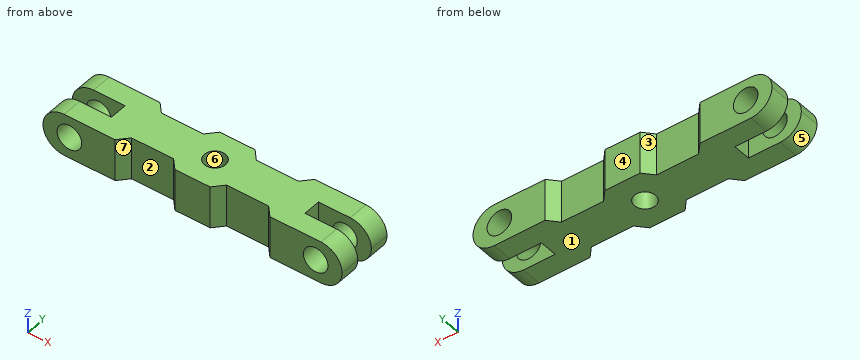
from build123d import *

# Parameters (mm, degrees)
F1_DEPTH = 12
F2_R     = 6
F3_DEPTH = 25
F4_R     = 7
F5_DEPTH = 50
F6_R     = 11.99999
F7_R     = 11.99999


# Not quite as in the source:
# - a fillet or chamfer is up to 0.001 mm smaller than in the source, because OpenCascade refuses the exact size


with BuildPart() as f1:
    # F0 (on Top) → F1 (new body, symmetric)
    with BuildSketch(Plane.XY):
        Polygon((10, 16.5), (0, 16.5), (-10, 16.5), (-15, 11), (-39, 11), (-44, 16.5), (-85, 16.5), (-85, 5), (-55, 5), (-55, 0), (-55, -5), (-85, -5), (-85, -16.5), (-44, -16.5), (-39, -11), (-15, -11), (-10, -16.5), (0, -16.5), (10, -16.5), (15, -11), (39, -11), (44, -16.5), (85, -16.5), (85, -5), (55, -5), (55, 0), (55, 5), (85, 5), (85, 16.5), (44, 16.5), (39, 11), (15, 11), align=None)
    extrude(amount=F1_DEPTH, both=True)

    # F2 (on Top) → F3 (cut, symmetric)
    with BuildSketch(Plane.XY):
        Circle(F2_R)
    extrude(amount=F3_DEPTH, both=True, mode=Mode.SUBTRACT)

    # F4 (on Front) → F5 (cut, symmetric)
    with BuildSketch(Plane.XZ):
        with Locations((70, 0)):
            Circle(F4_R)
        with Locations((-70, 0)):
            Circle(F4_R)
    extrude(amount=F5_DEPTH, both=True, mode=Mode.SUBTRACT)

    # F6 (radius 12 in the source; OpenCascade refuses exactly that, so slightly less here)
    f6_edges = [f1.edges().sort_by_distance(p)[0] for p in [
        (85, 10.75, 12),
        (85, -10.75, 12),
        (85, -10.75, -12),
        (85, 10.75, -12),
    ]]
    fillet(f6_edges, radius=F6_R)

    # F7 (radius 12 in the source; OpenCascade refuses exactly that, so slightly less here)
    f7_edges = [f1.edges().sort_by_distance(p)[0] for p in [
        (-85, -10.75, 12),
        (-85, 10.75, 12),
        (-85, 10.75, -12),
        (-85, -10.75, -12),
    ]]
    fillet(f7_edges, radius=F7_R)


solid = f1.part
Geometry check sheet. Reference: the model listing, model coordinates, mm. Face numbers are marked on the shaded views. A direction names the side the tool comes from. Round coordinates to 2 decimals unless told otherwise and drop trailing zeros. Loops run counter-clockwise (first coordinate to the right, second up) from the corner with the lowest first, then second, coordinate; pieces in that order, holes last.
Item 1: Mould release check, pull along Y, two halves, no side actions. Record for the marked faces 4, 5, 6 and 7: pulls with the +Y half, pulls with the -Y half, needs draft (parallel to the pull), parting line crosses it, or undercut.
Item 2: Cross-section at D-D on y = 0. Record the boundary of the cut face in (x, z).
Item 3: Thickness scan on line 1 (Y direction, x = 65.5, z = -7.25); line 2 (X direction, y = 8, z = 2.5); line 3 (Y direction, x = 0, z = 6.75). Record the ranges inside material, lowest first.
Item 4: Access from +Z, -Z, +X, -X, +Y, -Y to the whole of each face (thin tool, end or side, straight path). Record for the marked faces 1, 2 and 3.
Item 5: Cross-section at A-A on x = 0. Record the boundary of the cut face in (y, z).
Item 6: Cross-section at C-C on x = -70. Record the boundary of the cut face in (y, z).
Item 7: Gauge pin test, flat ends, axial feed: pin 1 (8.5 mm diameter, centred on x = 70, z = 0, fed in from +Y); pin 2 (19 mm diameter, centred on x = 0, y = 0, fed in from +Z); pin 3 (11 mm diameter, centred on y = 0.5, z = -5.5, fed in from +X); pin 4 (8 mm diameter, centred on y = -8, z = -6.5, fed in from -X). Record the tip position at first contact, or that the pin passes through.
Item 8: Cross-section at B-B on y = -9.5. Count the separate pieces of the cut face and the enclosed holes in it, then the cut area to 3 significant figures.
Answer sheet:
1. face 4: pulls with the +Y half
1. face 5: needs draft
1. face 6: undercut
1. face 7: pulls with the -Y half
2. outline: (-55, -12) - (-6, -12) - (-6, 12) - (-55, 12) - close; (6, -12) - (55, -12) - (55, 12) - (6, 12) - close
3. line 1: y = -16.5 to -5, 5 to 16.5
3. line 2: x = -84.74 to -76.54, -63.46 to 63.46, 76.54 to 84.74
3. line 3: y = -16.5 to -6, 6 to 16.5
4. face 1: -Z, +X, -X, +Y, -Y
4. face 2: +Z, -Z, -Y
4. face 3: +Z, -Z, +Y
5. outline: (-16.5, -12) - (-6, -12) - (-6, 12) - (-16.5, 12) - close; (6, -12) - (16.5, -12) - (16.5, 12) - (6, 12) - close
6. outline: (-16.5, -12) - (-5, -12) - (-5, -7) - (-16.5, -7) - close; (-16.5, 7) - (-5, 7) - (-5, 12) - (-16.5, 12) - close; (5, -12) - (16.5, -12) - (16.5, -7) - (5, -7) - close; (5, 7) - (16.5, 7) - (16.5, 12) - (5, 12) - close
7. pin 1: passes through
7. pin 2: stops at z = 12
7. pin 3: stops at x = 84.77
7. pin 4: stops at x = -84.74
8. separate pieces: 1
8. enclosed holes: 2
8. area: 3,650 mm2
